Can you work these out from the drawing? Everything is in mm from the part's minimum corner. Round coordinates to 2 decimals unless told otherwise and drop trailing zeros. Write each loop counter-clockwise with the first axis right and the second up, starting at its lowest first coordinate (ties: lowest second). Pieces come first, ordered by that corner, then holes. Notation, with made-up numbers: (-14, 8.25) -> (30, 8.25) arc R34 ccw to (30, 47.25) -> close; hole circle Ø3 at (47, 54). An arc over 180 degrees is marked (long way). Write item = value, one per line. Start each with the question number.
1) Imagine slicing it at A-A, the plane z = 10. Please give me the cut outline in (x, y), then the cut area to 3 significant figures.
2) Thinking about a two-plate mould opening in Z: for the marked faces 1, 2, 3 and 4, which applies, +Z half, -Z half, draft (parallel to the pull), parting line (faces both ways), or undercut?
3) Imagine slicing it at C-C, the plane y = 2.5. Please give me the cut outline in (x, z), then the cut area to 3 significant figures.
4) Imagine slicing it at B-B, the plane x = 0.75. Please give me the cut outline in (y, z).
5) Imagine slicing it at D-D, the plane x = 2.7. Please give me the cut outline in (y, z), then the cut area to 3 significant figures.
6) If I drill on line 1 (Z direction, x = 0.3, y = 4.6); line 2 (Z direction, x = 2.25, y = 2.5); line 3 (X direction, y = 2.55, z = 5.75), over which ranges is the centre line in solid material (lowest first)?
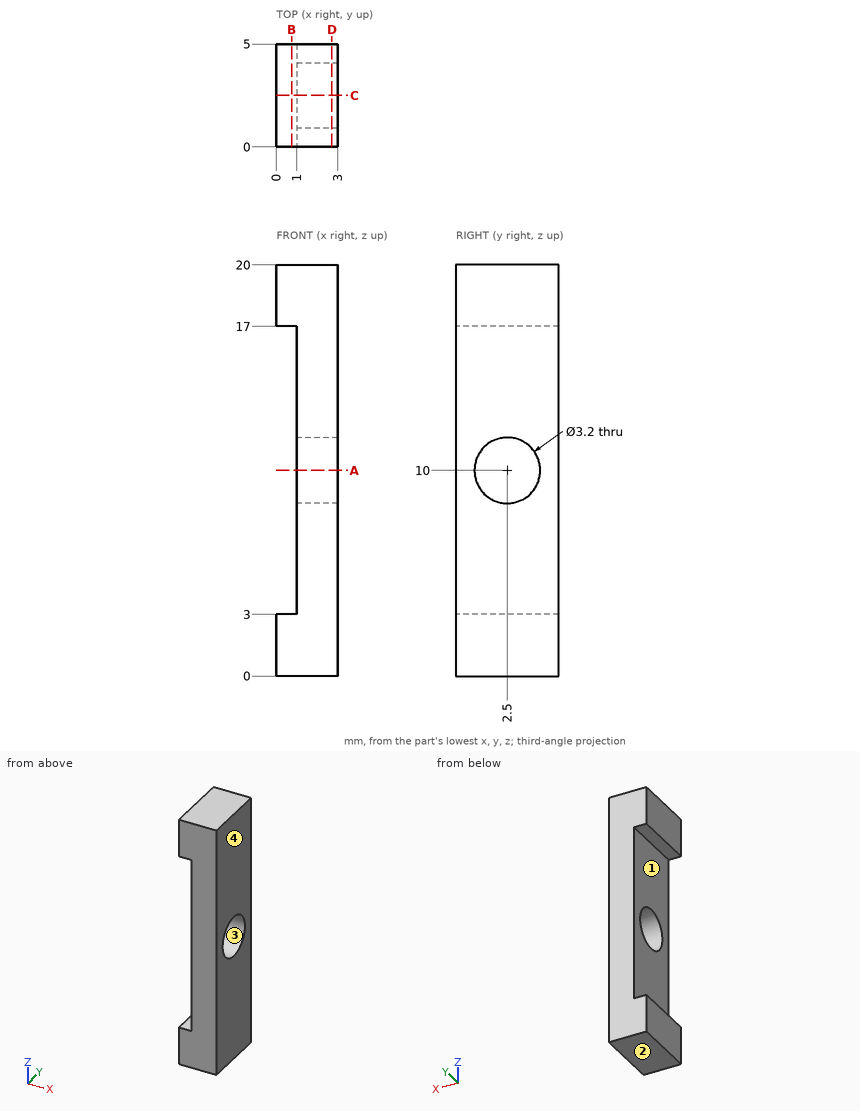
Reported:
q1.outline = (1, 0) -> (3, 0) -> (3, 0.9) -> (1, 0.9) -> close; (1, 4.1) -> (3, 4.1) -> (3, 5) -> (1, 5) -> close
q1.area = 3.60 mm²
q2.face_1 = undercut
q2.face_2 = -Z half
q2.face_3 = undercut
q2.face_4 = draft
q3.outline = (0, 0) -> (3, 0) -> (3, 8.4) -> (1, 8.4) -> (1, 3) -> (0, 3) -> close; (0, 17) -> (1, 17) -> (1, 11.6) -> (3, 11.6) -> (3, 20) -> (0, 20) -> close
q3.area = 39.6 mm²
q4.outline = (0, 0) -> (5, 0) -> (5, 3) -> (0, 3) -> close; (0, 17) -> (5, 17) -> (5, 20) -> (0, 20) -> close
q5.outline = (0, 0) -> (5, 0) -> (5, 20) -> (0, 20) -> close; hole circle Ø3.2 at (2.5, 10)
q5.area = 92.0 mm²
q6.line_1 = 0 to 3, 17 to 20
q6.line_2 = 0 to 8.4, 11.6 to 20
q6.line_3 = 1 to 3
